Autodesk Inventor part; units mm, degrees
ref_plane "Work Plane1" through (0, 16.51, 0) normal (0, 1, 0) x (-1, 0, 0)
ref_plane "YZ Plane" through (0, 0, 0) normal (1, 0, 0) x (0, 1, 0)
ref_plane "XY Plane" through (0, 0, 0) normal (0, 0, 1) x (1, 0, 0)
sketch "Sketch1" plane through (0, 0, 0) normal (0, 0, 1) x (1, 0, 0)
  line L0 (17.78, 17.78) -> (-17.78, 17.78)
  line L1 (-17.78, 17.78) -> (-17.78, -17.78)
  line L2 (-17.78, -17.78) -> (17.78, -17.78)
  line L3 (17.78, -17.78) -> (17.78, 17.78)
  point P0 (0, 0)
  dimension "d0" = 35.56
  dimension "d1" = 35.56
  dimension "d2" = 17.78
  dimension "d3" = 17.78
extrude "Extrusion1" add sketch "Sketch1" along normal blind 2.54
sketch "Sketch2" plane through (0, 0, 2.54) normal (0, 0, 1) x (1, 0, 0)
  circle A0 centre (0, 0) radius 12.7
  circle A1 centre (0, 0) radius 16.51
  dimension "d6" = 25.4
  dimension "d7" = 3.81
extrude "Extrusion2" add sketch "Sketch2" along normal blind 31.75
sketch "Sketch3" plane through (0, 0, 2.54) normal (0, 0, 1) x (1, 0, 0)
  line L0 (17.78, 17.78) -> (-17.78, 17.78)
  line L1 (-17.78, 17.78) -> (-17.78, -17.78)
  line L2 (17.78, -17.78) -> (17.78, 17.78)
  line L3 (-17.78, -17.78) -> (17.78, -17.78)
  point P0 (0, 0)
  point P1 (-13.97, -13.97)
  point P2 (13.97, -13.97)
  point P3 (13.97, 13.97)
  point P4 (-13.97, 13.97)
  dimension "d10" = 3.81
  dimension "d11" = 3.81
  dimension "d12" = 3.81
  dimension "d13" = 3.81
  dimension "d14" = 3.81
  dimension "d15" = 3.81
  dimension "d16" = 3.81
  dimension "d17" = 3.81
hole "Hole1" at (-13.97, -13.97, 2.54) at (13.97, -13.97, 2.54) at (13.97, 13.97, 2.54) at (-13.97, 13.97, 2.54) direction (0, 0, -1) diameter 3.175 depth 3.175 tip angle 118
ref_plane "Work Plane1" through (0, 16.51, 0) normal (0, 1, 0) x (-1, 0, 0)
sketch "Sketch4" plane through (0, 16.51, 0) normal (0, 1, 0) x (-1, 0, 0)
  line L0 (-12.7, 34.29) -> (12.7, 34.29)
  line L1 (5.08, 34.29) -> (-5.08, 34.29)
  line L2 (-5.08, 34.29) -> (-5.08, 29.21)
  line L3 (-5.08, 29.21) -> (5.08, 29.21)
  line L4 (5.08, 29.21) -> (5.08, 34.29)
  line L5 (0, -6.858) -> (0, 41.148)
  point P0 (0, 0)
  dimension "d26" = 5.08
  dimension "d27" = 10.16
  dimension "d28" = 5.08
extrude "Extrusion3" cut sketch "Sketch4" against normal blind 10.16
sketch "Sketch5" plane through (0, 0, 2.54) normal (0, 0, 1) x (1, 0, 0)
  circle A0 centre (0, 0) radius 4.445
  dimension "d31" = 8.89
extrude "Extrusion4" cut sketch "Sketch5" against normal through all
fillet "Fillet1" radius 1.27 4 edges at (-5.08, 13.6744, 29.21) (-5.08, 13.6744, 34.29) (5.08, 13.6744, 34.29) (5.08, 13.6744, 29.21)
properties part number "000114"
CAD build for the part. Positions are in the model's coordinates, mm. A direction names the side the tool comes from. Round coordinates to 2 decimals unless told otherwise and drop trailing zeros. Write each loop counter-clockwise with the first axis right and the second up, starting at its lowest first coordinate (ties: lowest second). Pieces come first, ordered by that corner, then holes.
(1) Drop flat-ended pins along their axis: P1, Ø5.5, axis at x = 0, y = 0, coming from the +Z side; P2, Ø20.5, axis at x = 0, y = 0, coming from the +Z side; P3, Ø4, axis at y = 7.5, z = 11.5, coming from the +X side; P4, Ø1.3, axis at x = 2, y = 13, coming from the +Z side. Give the stop position or say it passes through.
(2) Slice it at B-B, the plane x = -14.5. Write the cut outline in (y, z), and give its area (3 significant figures).
(3) Slice it at C-C, the plane y = 13.97. Write the cut outline in (x, z), and give its area (3 significant figures).
(4) Mould opens along Y. For faces 4 (the face through (-12.42, 14.31, 1.25)), 5 (the face through (0, -17.78, 1)), 6 (the face through (17.78, 0, 1)) say: pulls with the +Y half, pulls with the -Y half, needs draft (parallel to the pull), parting line crosses it, or undercut.
(5) Slice it at A-A, the plane y = 0. Write the cut outline in (x, z) (3 decimals).
(6) 3-axis set-ups, long thin cutter, end or side, ignore diameter. For faces 1 (the face through (-4.718, 13.821, 29.592)), 2 (the face through (-2.15, -16.37, 18.19)), 3 (the face through (0, 17.78, 1)): which of +Z, -Z, +X, -X, +Y, -Y reach the whole face in a straight line?
(7) Slice it at D-D, the plane x = -7.5. Write the cut outline in (y, z), and give its area (3 significant figures).
(8) Probe line 1 along X through (y, z) = (13.97, 1.5); line 2 along Y through (x, z) = (-0.5, 24). List the from-to ranges inside material, lowest first.
From the geometry:
1. P1: passes through
1. P2: stops at z = 2.54
1. P3: stops at x = 15.57
1. P4: stops at z = 29.21
2. outline: (-17.78, 0) - (-15.47, 0) - (-15.47, 2.54) - (-17.78, 2.54) - close; (-12.47, 0) - (12.47, 0) - (12.47, 2.54) - (7.89, 2.54) - (7.89, 34.29) - (-7.89, 34.29) - (-7.89, 2.54) - (-12.47, 2.54) - close; (15.47, 0) - (17.78, 0) - (17.78, 2.54) - (15.47, 2.54) - close
2. area: 576 mm2
3. outline: (-17.78, 0) - (-15.56, 0) - (-15.56, 2.54) - (-17.78, 2.54) - close; (-12.38, 0) - (12.38, 0) - (12.38, 2.54) - (8.8, 2.54) - (8.8, 34.29) - (6.35, 34.29) arc R1.27 ccw to (5.08, 33.02) - (5.08, 30.48) arc R1.27 cw to (3.81, 29.21) - (-3.81, 29.21) arc R1.27 cw to (-5.08, 30.48) - (-5.08, 33.02) arc R1.27 ccw to (-6.35, 34.29) - (-8.8, 34.29) - (-8.8, 2.54) - (-12.38, 2.54) - close; (15.56, 0) - (17.78, 0) - (17.78, 2.54) - (15.56, 2.54) - close
3. area: 581 mm2
4. face 4: undercut
4. face 5: pulls with the -Y half
4. face 6: needs draft
5. outline: (-17.78, 0) - (-4.445, 0) - (-4.445, 2.54) - (-12.7, 2.54) - (-12.7, 34.29) - (-16.51, 34.29) - (-16.51, 2.54) - (-17.78, 2.54) - close; (4.445, 0) - (17.78, 0) - (17.78, 2.54) - (16.51, 2.54) - (16.51, 34.29) - (12.7, 34.29) - (12.7, 2.54) - (4.445, 2.54) - close
6. face 1: +Z, +Y
6. face 2: +Z
6. face 3: +Z, -Z, +X, -X, +Y
7. outline: (-17.78, 0) - (17.78, 0) - (17.78, 2.54) - (14.71, 2.54) - (14.71, 34.29) - (10.25, 34.29) - (10.25, 2.54) - (-10.25, 2.54) - (-10.25, 34.29) - (-14.71, 34.29) - (-14.71, 2.54) - (-17.78, 2.54) - close
7. area: 373 mm2
8. line 1: x = -17.78 to -15.56, -12.38 to 12.38, 15.56 to 17.78
8. line 2: y = -16.5 to -12.69, 12.69 to 16.5
